Build history of the part. All positions in model axes, mm. A direction names the side the tool comes from. Give positions to 0.01 mm unless a question says otherwise; leave off trailing zeros. Put each result on its own line as item: value.
Autodesk Inventor part; units mm, degrees
ref_plane "YZ Plane" through (0, 0, 0) normal (1, 0, 0) x (0, 1, 0)
ref_plane "XZ Plane" through (0, 0, 0) normal (0, 1, 0) x (-1, 0, 0)
ref_plane "XY Plane" through (0, 0, 0) normal (0, 0, 1) x (1, 0, 0)
sketch "Skizze1" plane through (0, 0, 0) normal (0, 1, 0) x (-1, 0, 0)
  circle A0 centre (0, 0) radius 31.5
  circle A1 centre (0, 0) radius 26.5
  dimension "d0" = 63
  dimension "d1" = 53
extrude "Extrusion1" add sketch "Skizze1" along normal blind 1.5
sketch "Skizze2" plane through (0, 1.5, 0) normal (0, 1, 0) x (1, 0, 0)
  circle A0 centre (0, 0) radius 31.5
extrude "Extrusion2" add sketch "Skizze2" along normal blind 2
sketch "Skizze3" plane through (0, 3.5, 0) normal (0, 1, 0) x (1, 0, 0)
  circle A0 centre (0, 0) radius 31.5
  circle A1 centre (0, 0) radius 26.5
  dimension "d6" = 53
extrude "Extrusion3" add sketch "Skizze3" along normal blind 1.5
chamfer "Fase1" distance 1.5 angle 45 1 edges at (-26.5, 5, 0)
chamfer "Fase2" distance 1.5 angle 45 1 edges at (26.5, 0, 0)
properties part number "Puk"
1) Tool access for faces 1 (the flat face through (-21, 5, 19)), 2 (the flat face through (0, 1.5, 0)): list every direction of +Z, -Z, +X, -X, +Y, -Y with a clear straight run to the whole face (end or side of a thin tool).
Filled sheet:
face 1: +Z, -Z, +X, -X, +Y
face 2: -Y
2) Pin check, flat tips, straight feed: pin 1 (1.5 mm diameter, centred on y = 2, z = -19, fed in from +X); pin 2 (2 mm diameter, centred on x = -2, y = 2.5, fed in from +Z); pin 3 (5 mm diameter, centred on x = 14, z = -10.5, fed in from +Y). Stop position of each tip, or through.
Filled sheet:
pin 1: x = 25.67
pin 2: z = 31.48
pin 3: y = 3.5
3) Wall check: L1, parallel to X at y = 3.55, z = 0; L2, parallel to Z at x = 7.5, y = 4.75; L3, parallel to Y at x = 3, z = 19.5. Give the ranges that are in metal, low to high.
Filled sheet:
L1: -31.5 to -26.55, 26.55 to 31.5
L2: -30.59 to -26.72, 26.72 to 30.59
L3: 1.5 to 3.5
4) Pull direction X, two halves, no side cores. Call faces 3 (the flat face through (0, 3.5, 0)), 4 (the flat face through (21, 0, -19)): released by +X, released by -X, zero draft, split by the parting line, or undercut.
Filled sheet:
face 3: undercut
face 4: zero draft
